The listing builds one solid part. Answer for the finished solid, in the listing's coordinates (mm). A direction names the side the tool comes from. Round coordinates to 2 decimals unless told otherwise and drop trailing zeros. Write each loop counter-clockwise with the first axis right and the second up, starting at its lowest first coordinate (ties: lowest second). Pieces come first, ordered by that corner, then holes. Notation, with made-up numbers: (50, 79) - (59, 79) arc R28 cw to (59, 101) - close; hole circle Ø4 at (47.25, -11). An arc over 180 degrees is marked (long way). Use a Markdown table: item, result. Add a question column.
1) A cutting plane is placed at B-B (y = 0). Give the vertices of the cut face in (x, z).
2) Each of these flat-tipped pins is pushed along its axis until it touches: P1, Ø14, axis at x = 70, y = 0, coming from the +Z side; P2, Ø3, axis at y = 24.5, z = 21, coming from the +X side; P3, Ø1.3, axis at x = -7, z = 53.5, coming from the +Y side; P4, Ø4, axis at x = 74, z = 22.5, coming from the -Y side. Where does it stop, or does it pass through?
3) A tool of negligible diameter and unlimited length cuts with its end or side. For faces 1 (the flat face through (-1, 25.629, 37)), 2 (the flat face through (20, -20, 0)), 3 (the cylindrical face through (20.765, -39.923, 47.157)), from which of +Z, -Z, +X, -X, +Y, -Y can it reach the whole face along a straight path? Write none if from no direction.
4) Find the intervals of material crossed by probe 1 along Z at (x, y) = (-3, -48); probe 2 along Y at (x, z) = (2.5, 48.5); probe 3 along Y at (x, z) = (0, 32), in increasing order. Write a range as from..to.
5) A cutting plane is placed at D-D (z = 32). Give the vertices of the cut face in (x, y).
6) A cutting plane is placed at C-C (z = 14.5). Give the vertices of the cut face in (x, y).
7) Determine the mould class of faces 4 (the cylindrical face through (-20.59, -92.74, 8.38)), 5 (the flat face through (18, -18, 75)), 6 (the cylindrical face through (0.9, -22.48, 36.98)) for opening direction Y: +Y half, -Y half, draft (parallel to the pull), parting line (faces both ways), or undercut.
8) A cutting plane is placed at A-A (x = 0). Give the vertices of the cut face in (y, z).
```python
from build123d import *

# Parameters (mm, degrees)
SKETCH2_R           = 95
BOSS_EXTRUDE1_DEPTH = 20
SKETCH3_R           = 45
BOSS_EXTRUDE2_DEPTH = 55
SKETCH4_R           = 22.5
CUT_EXTRUDE1_DEPTH  = 75
SKETCH5_R           = 6
CUT_EXTRUDE2_DEPTH  = 20
SKETCH6_W           = 14
SKETCH6_H           = 4
CUT_EXTRUDE3_DEPTH  = 75
FILLET1_R           = 3


with BuildPart() as part:
    # Sketch2 → Boss-Extrude1 (new body)
    with BuildSketch(Plane.XY):
        Circle(SKETCH2_R)
    extrude(amount=BOSS_EXTRUDE1_DEPTH)

    # Sketch3 → Boss-Extrude2 (add)
    with BuildSketch(Plane.XY.offset(20)):
        Circle(SKETCH3_R)
    extrude(amount=BOSS_EXTRUDE2_DEPTH)

    # Sketch4 → Cut-Extrude1 (cut)
    with BuildSketch(Plane(origin=(0, 0, 0), x_dir=(-1, 0, 0), z_dir=(0, 0, -1))):
        Circle(SKETCH4_R)
    extrude(amount=-CUT_EXTRUDE1_DEPTH, mode=Mode.SUBTRACT)

    # Sketch5 → Cut-Extrude2 (cut)
    with BuildSketch(Plane(origin=(0, 0, 0), x_dir=(-1, 0, 0), z_dir=(0, 0, -1))):
        with Locations((0, 70)):
            Circle(SKETCH5_R)
        with Locations((70, 0)):
            Circle(SKETCH5_R)
        with Locations((0, -70)):
            Circle(SKETCH5_R)
        with Locations((-70, 0)):
            Circle(SKETCH5_R)
    extrude(amount=-CUT_EXTRUDE2_DEPTH, mode=Mode.SUBTRACT)

    # Sketch6 → Cut-Extrude3 (cut)
    with BuildSketch(Plane(origin=(0, 0, 0), x_dir=(-1, 0, 0), z_dir=(0, 0, -1))):
        with Locations((0.80166167, 23.629392085)):
            Rectangle(SKETCH6_W, SKETCH6_H)
    extrude(amount=-CUT_EXTRUDE3_DEPTH, mode=Mode.SUBTRACT)

    # Fillet1
    fillet1_edges = [part.edges().sort_by_distance(p)[0] for p in [
        (-95, 0, 20),
        (-45, 0, 20),
        (-45, 0, 75),
    ]]
    fillet(fillet1_edges, radius=FILLET1_R)


solid = part.part
```
Entries:
| question | item | result |
|---|---|---|
| 1 | outline | (-95, 0) - (-76, 0) - (-76, 20) - (-92, 20) arc R3 ccw to (-95, 17) - close; (-64, 0) - (-22.5, 0) - (-22.5, 75) - (-42, 75) arc R3 ccw to (-45, 72) - (-45, 23) arc R3 cw to (-48, 20) - (-64, 20) - close; (22.5, 0) - (64, 0) - (64, 20) - (48, 20) arc R3 cw to (45, 23) - (45, 72) arc R3 ccw to (42, 75) - (22.5, 75) - close; (76, 0) - (95, 0) - (95, 17) arc R3 ccw to (92, 20) - (76, 20) - close |
| 2 | P1 | stops at z = 20 |
| 2 | P2 | stops at x = 90.43 |
| 2 | P3 | stops at y = 44.55 |
| 2 | P4 | passes through |
| 3 | face 1 | +Z, -Z |
| 3 | face 2 | -Z, +X, -X, +Y, -Y |
| 3 | face 3 | +Z |
| 4 | probe 1 | z = 0..20 |
| 4 | probe 2 | y = -44.93..-22.36, 25.63..44.93 |
| 4 | probe 3 | y = -45..-22.5, 25.63..45 |
| 5 | outline | circle Ø90 at (0, 0); hole (-7.8, 21.63) - (-6.2, 21.63) arc R22.5 ccw (long way) to (6.2, 21.63) - (6.2, 25.63) - (-7.8, 25.63) - close |
| 6 | outline | circle Ø190 at (0, 0); hole circle Ø12 at (-70, 0); hole (-7.8, 21.63) - (-6.2, 21.63) arc R22.5 ccw (long way) to (6.2, 21.63) - (6.2, 25.63) - (-7.8, 25.63) - close; hole circle Ø12 at (0, -70); hole circle Ø12 at (0, 70); hole circle Ø12 at (70, 0) |
| 7 | face 4 | parting line |
| 7 | face 5 | draft |
| 7 | face 6 | undercut |
| 8 | outline | (-95, 0) - (-76, 0) - (-76, 20) - (-92, 20) arc R3 ccw to (-95, 17) - close; (-64, 0) - (-22.5, 0) - (-22.5, 75) - (-42, 75) arc R3 ccw to (-45, 72) - (-45, 23) arc R3 cw to (-48, 20) - (-64, 20) - close; (25.63, 0) - (64, 0) - (64, 20) - (48, 20) arc R3 cw to (45, 23) - (45, 72) arc R3 ccw to (42, 75) - (25.63, 75) - close; (76, 0) - (95, 0) - (95, 17) arc R3 ccw to (92, 20) - (76, 20) - close |
